The listing builds one solid part. Answer for the finished solid, in the listing's coordinates (mm). A direction names the side the tool comes from. Round coordinates to 2 decimals unless told otherwise and drop trailing zeros. Order: outer loops, then holes, each group sorted by start corner. A loop starts at its lowest first (then second) coordinate and runs counter-clockwise, first axis right, second up. Notation, with made-up numbers: (64, 76.5) - (103, 76.5) arc R35 cw to (103, 112.5) - close; hole circle Ø11 at (79, -8.75). An arc over 180 degrees is marked (long way). One line per item, written item: value. Start each with the question number.
1. Flat-ended cylindrical pins translate along their axes: P1, Ø8, axis at x = -14, z = -6, coming from the -Y side; P2, Ø3, axis at y = 2, z = 28, coming from the -X side; P3, Ø6, axis at x = -5, y = 1, coming from the -Z side; P4, Ø2, axis at y = -4.28, z = 48.9, coming from the +X side. Find the tip coordinate at first contact, or state that the pin passes through.
2. A tool of negligible diameter and unlimited length cuts with its end or side. For faces 1 (the flat face through (-4.826, -2, 45)), 2 (the cylindrical face through (16.38, 3.13, 36.5)), 3 (the cylindrical face through (-8.18, 2, 36.82)), from which of +Z, -Z, +X, -X, +Y, -Y can it reach the whole face along a straight path? Write none if from no direction.
3. Section D-D, the plane x = -22.5 is taken. Give the vertices of the cut face in (y, z).
4. Section C-C, the plane y = -8 is taken. Give the vertices of the cut face in (x, z).
5. Section A-A, the plane z = 0 is taken. Give the vertices of the cut face in (x, y) (3 decimals), then the cut area to 3 significant figures.
6. Straight lines are drawn through the part: line 1 (X direction, y = 2.3, z = 0) (3 decimals); line 2 (Y direction, x = -14, z = 37); line 3 (Y direction, x = -19, z = -34). For each, find the intervals that lie inside material, in ascending order.
7. For a pull along Y with two mould halves and no side action, classify faces 4 (the flat face through (-1, 6.35, 1)), 5 (the flat face through (4.826, -2, 45)), 6 (the flat face through (-1, 4.064, -1)), 7 (the cylindrical face through (-0.068, -5.423, 49.499)) as released by +Y, released by -Y, zero draft, split by the parting line, or undercut.
8. Section B-B, the plane x = 0 is taken. Give the vertices of the cut face in (y, z) (3 decimals).
from build123d import *

# Parameters (mm, degrees)
SKETCH1_R           = 40.005
BOSS_EXTRUDE1_DEPTH = 6.35
BOSS_EXTRUDE2_DEPTH = 2.54
SHELL2_OUTLINE_R    = 37.719
SHELL2_DEPTH        = 4.064
SHELL2_2_DEPTH      = 0.254
BOSS_EXTRUDE3_DEPTH = 4.826
CUT_EXTRUDE1_REACH  = 70.416
SKETCH10_R          = 1.293229199


# Read off the part's stored shape, not the designer's step: Shell2
with BuildPart() as part:
    # Sketch1 → Boss-Extrude1 (new body)
    with BuildSketch(Plane(origin=(0, 0, 0), x_dir=(1, 0, 0), z_dir=(0, 1, 0))):
        with Locations(Location((0, 0, 0), (0, 0, 270))):
            Circle(SKETCH1_R)
    extrude(amount=BOSS_EXTRUDE1_DEPTH)

    # Sketch2 → Boss-Extrude2 (add)
    with BuildSketch(Plane(origin=(0, 0, 0), x_dir=(1, 0, 0), z_dir=(0, 1, 0))):
        with BuildLine():
            ThreePointArc((-36.439263508, 16.51), (0, 49.926276753), (36.439263508, 16.51))
            ThreePointArc((36.439263508, 16.51), (0, -40.005), (-36.439263508, 16.51))
        make_face()
    extrude(amount=BOSS_EXTRUDE2_DEPTH)

    # Shell2 outline → Shell2 (cut)
    with BuildSketch(Plane(origin=(0, 0, 0), x_dir=(1, 0, 0), z_dir=(0, 1, 0))):
        Circle(SHELL2_OUTLINE_R)
    extrude(amount=SHELL2_DEPTH, mode=Mode.SUBTRACT)

    # Shell2 2 outline → Shell2 2 (cut)
    with BuildSketch(Plane(origin=(0, 0, 0), x_dir=(1, 0, 0), z_dir=(0, 1, 0))):
        with BuildLine():
            ThreePointArc((-34.19336189, 15.922844082), (0, 37.719), (34.19336189, 15.922844082))
            ThreePointArc((34.19336189, 15.922844082), (0, 47.640276753), (-34.19336189, 15.922844082))
        make_face()
    extrude(amount=SHELL2_2_DEPTH, mode=Mode.SUBTRACT)



with BuildPart() as body_2:
    # Sketch6 → Boss-Extrude3 (new, symmetric)
    with BuildSketch(Plane(origin=(0, 0, 0), x_dir=(0, 0, -1), z_dir=(1, 0, 0))):
        Polygon((-40.005, 6.35), (-50.673, 0), (-50.673, -10.16), (-46.228, -10.16), (-46.228, -3.81), (-40.005, 0), align=None)
    extrude(amount=BOSS_EXTRUDE3_DEPTH, both=True)


with BuildPart() as part_1:
    add(part.part)

    add(body_2.part)  # Loft1 merges body 2
    # Sketch9 → Loft1 section 0
    with BuildSketch(Plane.XY.offset(38.1)):
        with BuildLine():
            Line((-5.008565366, 6.35), (5.151434634, 6.35))
            Line((5.151434634, 6.35), (5.151434634, 0))
            Line((5.151434634, 0), (-5.008565366, 0))
            Line((-5.008565366, 0), (-5.008565366, 6.35))
        make_face()
    # Sketch7 → Loft1 section 1
    with BuildSketch(Plane(origin=(0, 0, 40.005), x_dir=(-1, 0, 0), z_dir=(0, 0, -1))):
        with BuildLine():
            Line((-5.151434634, 0), (5.008565366, 0))
            Line((5.008565366, 0), (5.008565366, 6.35))
            Line((5.008565366, 6.35), (-5.151434634, 6.35))
            Line((-5.151434634, 6.35), (-5.151434634, 0))
        make_face()
    loft()

    # Sketch10 → Cut-Extrude1 (cut, up to next)
    with BuildSketch(Plane.ZY.offset(4.826), mode=Mode.PRIVATE) as cut_extrude1_sk1:
        with Locations((48.902107894, -4.275925595)):
            Circle(SKETCH10_R)
    cut_extrude1_tool1 = extrude(cut_extrude1_sk1.sketch, amount=-CUT_EXTRUDE1_REACH, mode=Mode.PRIVATE) & part_1.part
    add(cut_extrude1_tool1.solids().sort_by_distance((-4.826, -4.275926, 48.902108))[0], mode=Mode.SUBTRACT)


solid = part_1.part
Answer list:
1. P1: stops at y = 4.06
1. P2: stops at x = -29.97
1. P3: stops at z = -49.87
1. P4: passes through
2. face 1: +Z, -X, +Y, -Y
2. face 2: +Y
2. face 3: -Y
3. outline: (0, -42.19) - (2.54, -42.19) - (2.54, -33.08) - (6.35, -33.08) - (6.35, 33.08) - (0, 33.08) - (0, 30.27) - (4.06, 30.27) - (4.06, -30.27) - (0.25, -30.27) - (0.25, -39.23) - (0, -39.23) - close
4. outline: (-4.83, 46.23) - (4.83, 46.23) - (4.83, 50.67) - (-4.83, 50.67) - close
5. outline: (-40.005, 0) - (-37.719, 0) - (-37.719, 4.064) - (37.719, 4.064) - (37.719, 0) - (40.005, 0) - (40.005, 6.35) - (-40.005, 6.35) - close
5. area: 201 mm²
6. line 1: x = -40.005 to -37.719, 37.719 to 40.005
6. line 2: y = 0 to 6.35
6. line 3: y = 0.25 to 6.35
7. face 4: released by +Y
7. face 5: zero draft
7. face 6: released by -Y
7. face 7: undercut
8. outline: (-10.16, 46.228) - (-3.81, 46.228) - (0, 40.005) - (0, 37.719) - (4.064, 37.719) - (4.064, -37.719) - (0.254, -37.719) - (0.254, -47.64) - (0, -47.64) - (0, -49.926) - (2.54, -49.926) - (2.54, -40.005) - (6.35, -40.005) - (6.35, 40.005) - (0, 50.673) - (-10.16, 50.673) - close; hole circle Ø2.586 at (-4.276, 48.902)
